from build123d import *

# Parameters (mm, degrees)
SKETCH1_W                = 8
SKETCH1_H                = 7.2
BOSS_EXTRUDE1_DEPTH      = 3
CUT_EXTRUDE1_DEPTH       = 2
SKETCH3_R                = 0.49811532
CUT_EXTRUDE2_DEPTH       = 2
BOSS_EXTRUDE2_DEPTH      = 1
BOSS_EXTRUDE3_DEPTH      = 1
MIRROR22_COPY_1_SKETCH_W = 8
MIRROR22_COPY_1_SKETCH_H = 7.2
MIRROR22_COPY_1_DEPTH    = 3
MIRROR22_COPY_2_DEPTH    = 2
MIRROR22_COPY_3_SKETCH_R = 0.49811532
MIRROR22_COPY_3_DEPTH    = 2
MIRROR22_COPY_4_DEPTH    = 1
MIRROR22_COPY_5_DEPTH    = 1
MIRROR22_COPY_6_DEPTH    = 1
MIRROR22_COPY_7_DEPTH    = 1
FILLET6_R                = 0.5


with BuildPart() as part:
    # Sketch1 → Boss-Extrude1 (new body)
    with BuildSketch(Plane(origin=(0, 0, 0), x_dir=(1, 0, 0), z_dir=(0, 1, 0))):
        with Locations((4, -3.6)):
            Rectangle(SKETCH1_W, SKETCH1_H)
    boss_extrude1 = extrude(amount=BOSS_EXTRUDE1_DEPTH)

    # Sketch2 → Cut-Extrude1 (cut)
    with BuildSketch(Plane(origin=(0, 3, 0), x_dir=(1, 0, 0), z_dir=(0, 1, 0))):
        with BuildLine():
            Line((3.75, -1.5), (4.4, -1.5))
            ThreePointArc((4.4, -1.5), (6.65, -3.75), (4.4, -6))
            Line((4.4, -6), (3.75, -6))
            ThreePointArc((3.75, -6), (1.5, -3.75), (3.75, -1.5))
        make_face()
    cut_extrude1 = extrude(amount=-CUT_EXTRUDE1_DEPTH, mode=Mode.SUBTRACT)

    # Sketch3 → Cut-Extrude2 (cut, through all)
    with BuildSketch(Plane(origin=(0, 1, 0), x_dir=(1, 0, 0), z_dir=(0, 1, 0))):
        with Locations((2.7875, -3.75)):
            Circle(SKETCH3_R)
        with Locations((5.3625, -3.75)):
            Circle(SKETCH3_R)
    cut_extrude2 = extrude(amount=-CUT_EXTRUDE2_DEPTH, mode=Mode.SUBTRACT)

    # Sketch4 → Boss-Extrude2 (add)
    with BuildSketch(Plane.ZY):
        Polygon((0, 3), (0, 15.5), (3, 15.5), (7.2, 3), align=None)
    boss_extrude2 = extrude(amount=-BOSS_EXTRUDE2_DEPTH)

    # Sketch7 → Boss-Extrude3 (add)
    with BuildSketch(Plane(origin=(0, 0, 0), x_dir=(-1, 0, 0), z_dir=(0, 0, -1))):
        Polygon((0, 15.5), (-3, 15.5), (-8, 3), (0, 3), align=None)
    boss_extrude3 = extrude(amount=-BOSS_EXTRUDE3_DEPTH)

    # Mirror16: Boss-Extrude1, Cut-Extrude1, Cut-Extrude2, Boss-Extrude2, Boss-Extrude3 across plane
    add(boss_extrude1.mirror(Plane(origin=(0, 3, 0), x_dir=(0, 0, 1), z_dir=(1, 0, 0))))
    add(cut_extrude1.mirror(Plane(origin=(0, 3, 0), x_dir=(0, 0, 1), z_dir=(1, 0, 0))), mode=Mode.SUBTRACT)
    add(cut_extrude2.mirror(Plane(origin=(0, 3, 0), x_dir=(0, 0, 1), z_dir=(1, 0, 0))), mode=Mode.SUBTRACT)
    add(boss_extrude2.mirror(Plane(origin=(0, 3, 0), x_dir=(0, 0, 1), z_dir=(1, 0, 0))))
    add(boss_extrude3.mirror(Plane(origin=(0, 3, 0), x_dir=(0, 0, 1), z_dir=(1, 0, 0))))

    # Mirror21: Boss-Extrude1, Cut-Extrude1, Cut-Extrude2, Boss-Extrude2, Boss-Extrude3 across plane
    add(boss_extrude1.mirror(Plane(origin=(0, 3, 0), x_dir=(1, 0, 0), z_dir=(0, 0, 1))))
    add(cut_extrude1.mirror(Plane(origin=(0, 3, 0), x_dir=(1, 0, 0), z_dir=(0, 0, 1))), mode=Mode.SUBTRACT)
    add(cut_extrude2.mirror(Plane(origin=(0, 3, 0), x_dir=(1, 0, 0), z_dir=(0, 0, 1))), mode=Mode.SUBTRACT)
    add(boss_extrude2.mirror(Plane(origin=(0, 3, 0), x_dir=(1, 0, 0), z_dir=(0, 0, 1))))
    add(boss_extrude3.mirror(Plane(origin=(0, 3, 0), x_dir=(1, 0, 0), z_dir=(0, 0, 1))))

    # Mirror22: Boss-Extrude1, Cut-Extrude1, Cut-Extrude2 across plane
    add(boss_extrude1.mirror(Plane(origin=(0, 3, 0), x_dir=(0, 0, 1), z_dir=(-1, 0, 0))))
    add(cut_extrude1.mirror(Plane(origin=(0, 3, 0), x_dir=(0, 0, 1), z_dir=(-1, 0, 0))), mode=Mode.SUBTRACT)
    add(cut_extrude2.mirror(Plane(origin=(0, 3, 0), x_dir=(0, 0, 1), z_dir=(-1, 0, 0))), mode=Mode.SUBTRACT)

    # Mirror22 copy 1 sketch → Mirror22 copy 1 (add)
    with BuildSketch(Plane(origin=(0, 0, 0), x_dir=(-1, 0, 0), z_dir=(0, 1, 0))):
        with Locations((4, -3.6)):
            Rectangle(MIRROR22_COPY_1_SKETCH_W, MIRROR22_COPY_1_SKETCH_H)
    extrude(amount=MIRROR22_COPY_1_DEPTH)

    # Mirror22 copy 2 sketch → Mirror22 copy 2 (cut)
    with BuildSketch(Plane(origin=(0, 3, 0), x_dir=(-1, 0, 0), z_dir=(0, 1, 0))):
        with BuildLine():
            Line((3.75, -1.5), (4.4, -1.5))
            ThreePointArc((4.4, -1.5), (6.65, -3.75), (4.4, -6))
            Line((4.4, -6), (3.75, -6))
            ThreePointArc((3.75, -6), (1.5, -3.75), (3.75, -1.5))
        make_face()
    extrude(amount=-MIRROR22_COPY_2_DEPTH, mode=Mode.SUBTRACT)

    # Mirror22 copy 3 sketch → Mirror22 copy 3 (cut, through all)
    with BuildSketch(Plane(origin=(0, 1, 0), x_dir=(-1, 0, 0), z_dir=(0, 1, 0))):
        with Locations((2.7875, -3.75)):
            Circle(MIRROR22_COPY_3_SKETCH_R)
        with Locations((5.3625, -3.75)):
            Circle(MIRROR22_COPY_3_SKETCH_R)
    extrude(amount=-MIRROR22_COPY_3_DEPTH, mode=Mode.SUBTRACT)

    # Mirror22 copy 4 sketch → Mirror22 copy 4 (add)
    with BuildSketch(Plane(origin=(0, 0, 0), x_dir=(0, 0, -1), z_dir=(1, 0, 0))):
        Polygon((0, 3), (0, 15.5), (3, 15.5), (7.2, 3), align=None)
    extrude(amount=-MIRROR22_COPY_4_DEPTH)

    # Mirror22 copy 5 sketch → Mirror22 copy 5 (add)
    with BuildSketch(Plane.XY):
        Polygon((0, 15.5), (-3, 15.5), (-8, 3), (0, 3), align=None)
    extrude(amount=-MIRROR22_COPY_5_DEPTH)

    # Mirror22 copy 6 sketch → Mirror22 copy 6 (add)
    with BuildSketch(Plane(origin=(0, 0, 0), x_dir=(0, 0, 1), z_dir=(1, 0, 0))):
        Polygon((0, -3), (0, -15.5), (3, -15.5), (7.2, -3), align=None)
    extrude(amount=-MIRROR22_COPY_6_DEPTH)

    # Mirror22 copy 7 sketch → Mirror22 copy 7 (add)
    with BuildSketch(Plane(origin=(0, 0, 0), x_dir=(1, 0, 0), z_dir=(0, 0, -1))):
        Polygon((0, -15.5), (-3, -15.5), (-8, -3), (0, -3), align=None)
    extrude(amount=-MIRROR22_COPY_7_DEPTH)

    # Fillet6
    fillet6_edges = [part.edges().sort_by_distance(p)[0] for p in [
        (-1, 15.5, 2),
        (-2, 15.5, 1),
        (-3, 15.5, 0),
        (0, 15.5, -3),
        (1, 15.5, -2),
        (2, 15.5, -1),
        (-1, 15.5, -2),
        (-2, 15.5, -1),
        (1, 15.5, 2),
        (0, 15.5, 3),
        (2, 15.5, 1),
        (3, 15.5, 0),
    ]]
    fillet(fillet6_edges, radius=FILLET6_R)


solid = part.part
Model file for the job. Use its own axes, mm. A direction names the side the tool comes from. Give positions to 0.01 mm unless a question says otherwise; leave off trailing zeros. Order: outer loops, then holes, each group sorted by start corner. A loop starts at its lowest first (then second) coordinate and runs counter-clockwise, first axis right, second up. Notation, with made-up numbers: (59.25, 49) - (109.25, 49) arc R11 ccw to (109.25, 62) - close; hole circle Ø4 at (73, 65). An arc over 180 degrees is marked (long way). Return JSON: item names as keys, results as strings.
1) Flat gauge pins, fed straight in: P1, Ø1.9, axis at y = 9.5, z = -4, coming from the -X side; P2, Ø3.5, axis at x = -5, y = 8.5, coming from the -Z side; P3, Ø8, axis at y = 11.5, z = -0.5, coming from the -X side. Where does each tip first touch, or does it go through?
Geometry says:
{"P1": "x = -1", "P2": "z = -1", "P3": "x = -6.2"}
2) Cut at A-A, the plane y = 1.75. Give the cut face in (x, z).
Geometry says:
{"outline": "(-8, -7.2) - (8, -7.2) - (8, 7.2) - (-8, 7.2) - close; hole (-4.4, -6) - (-3.75, -6) arc R2.25 ccw to (-3.75, -1.5) - (-4.4, -1.5) arc R2.25 ccw to start; hole (-4.4, 1.5) - (-3.75, 1.5) arc R2.25 ccw to (-3.75, 6) - (-4.4, 6) arc R2.25 ccw to start; hole (3.75, -6) - (4.4, -6) arc R2.25 ccw to (4.4, -1.5) - (3.75, -1.5) arc R2.25 ccw to start; hole (3.75, 1.5) - (4.4, 1.5) arc R2.25 ccw to (4.4, 6) - (3.75, 6) arc R2.25 ccw to start"}
3) Pull direction Z, two halves, no side cores. Call faces 4 (the flat face through (4, 8, -1)), 5 (the flat face through (-5.2, 3, -6.1)), 6 (the flat face through (0, 1, 7.2)), 7 (the cylindrical face through (-1.5, 2, -3.8)): pulls with the +Z half, pulls with the -Z half, needs draft (parallel to the pull), parting line crosses it, or undercut.
Geometry says:
{"face 4": "pulls with the -Z half", "face 5": "needs draft", "face 6": "pulls with the +Z half", "face 7": "undercut"}
4) Cut at B-B, the plane z = -3.75. Count the separate pieces of the cut face and the enclosed holes in it, plus the area to 3 significant figures.
Geometry says:
{"separate pieces": "5", "enclosed holes": "0", "area": "44.0 mm²"}
5) Cut at D-D, the plane x = 0.25. Give the cut face in (y, z).
Geometry says:
{"outline": "(0, -7.2) - (3, -7.2) - (15.16, -3.11) arc R0.5 ccw to (15.5, -2.64) - (15.5, 2.64) arc R0.5 ccw to (15.16, 3.11) - (3, 7.2) - (0, 7.2) - close"}
6) Probe line 1 (Z direction, x = 4, y = 2); line 2 (X direction, y = 0.3, z = 3.75); line 3 (Z direction, x = -1.75, y = 7.75). List the from-to ranges inside material, lowest first. Write a range as from..to.
Geometry says:
{"line 1": "-7.2..-6, -1.5..1.5, 6..7.2", "line 2": "-8..-5.86, -4.86..-3.29, -2.29..2.29, 3.29..4.86, 5.86..8", "line 3": "-1..1"}
7) Cut at C-C, the plane z = 0. Give the cut face in (x, y).
Geometry says:
{"outline": "(-8, 0) - (8, 0) - (8, 3) - (3.13, 15.19) arc R0.5 ccw to (2.66, 15.5) - (-2.66, 15.5) arc R0.5 ccw to (-3.13, 15.19) - (-8, 3) - close"}
8) 3-axis set-ups, long thin cutter, end or side, ignore diameter. For faces 1 (the flat face through (-4, 1, -4)), 2 (the flat face through (0, 1, -7.2)), 3 (the flat face through (4, 8, 1)): which of +Z, -Z, +X, -X, +Y, -Y reach the whole face in a straight line?
Geometry says:
{"face 1": "+Y", "face 2": "-Z, +X, -X, +Y, -Y", "face 3": "+Z, +X, +Y"}
